For this review, take the finished solid that the model builds, in its own axes (mm). A direction names the side the tool comes from. Coordinates: 2 decimals unless noted, no trailing zeros. Loops run counter-clockwise (first coordinate to the right, second up) from the corner with the lowest first, then second, coordinate; pieces in that order, holes last. Notation, with made-up numbers: (87, -16) - (94, -16) arc R21 cw to (94, -1) - close; hole circle Ø7 at (57, -3.75). An arc over 180 degrees is marked (long way). One line per item, written item: value. Start each with the question number.
1. For faces 5 (the face through (-41.503, 6.12, -0.154)), 6 (the face through (-22.76, 3.595, 40.954)), 7 (the face through (42, 1.5, 7)), list the 3-axis set-ups (+Z, -Z, +X, -X, +Y, -Y) from which the entire face can be reached by the end or side of a thin tool; tool diameter is ignored.
2. To check wall thickness, follow line 1 (Z direction, x = -22.5, y = 6.1); line 2 (Z direction, x = 0, y = 0.75). State the ranges of each line that lie inside material, in increasing order. Write a range as from..to.
3. Take a section at A-A, the plane z = 0. Count the separate pieces of the cut face and the enclosed holes in it, and give its area (3 significant figures).
4. Insertion check: pin 1 (7.5 mm diameter, centred on x = -45, z = 0, fed in from +Y); pin 2 (3 mm diameter, centred on x = 25.5, y = 9, fed in from +Z); pin 3 (3.5 mm diameter, centred on x = -21, z = -39.5, fed in from +Y). Each pin has a flat end and moves straight along its axis. Give the tip position at first contact, or say it passes through.
5. Take a section at C-C, the plane x = 0. State the section outline as (y, z) points.
6. Take a section at D-D, the plane z = -12. State the section outline as (x, y) points, and give its area (3 significant figures).
7. The part is to be moulded in two halves that separate along Z. For faces 1 (the face through (-34, 6.5, -21)), 2 (the face through (-51, 4, 0)), 3 (the face through (43, 4, 0)), 4 (the face through (20, 5.75, -40)), say which applies: released by +Z, released by -Z, zero draft, split by the parting line, or undercut.
8. Take a section at B-B, the plane x = 45. State the section outline as (y, z) points, and give its area (3 significant figures).
```python
from build123d import *

# Parameters (mm, degrees)
EXTRUDE_1_DEPTH          = 5
PATTERN_CIRCULAR_1_COUNT = 6


with BuildPart() as part:
    # 草圖1 → 旋轉1 (revolve)
    with BuildSketch(Plane.XY):
        with BuildLine():
            Line((39.811273529, 6.5), (47.5, 6.5))
            Line((47.5, 6.5), (47.5, 1.5))
            Line((47.5, 1.5), (42, 1.5))
            Line((42, 1.5), (42, 0))
            Line((42, 0), (40, 0))
            Line((40, 0), (40, 0.927925359))
            ThreePointArc((40, 0.927925359), (22.903465984, 17.291823131), (0, 23.25))
            Line((0, 23.25), (0, 26.25))
            ThreePointArc((0, 26.25), (22.220486043, 21.041182168), (39.811273529, 6.5))
        make_face()
    revolve(axis=Axis((0, 0, 0), (0, 1, 0)))

    # 草圖3 → 填料-伸長1 (add)
    with BuildSketch(Plane(origin=(0, 6.5, 0), x_dir=(1, 0, 0), z_dir=(0, 1, 0))):
        with BuildLine():
            ThreePointArc((44.6, 5.986651819), (51, 0), (44.6, -5.986651819))
            ThreePointArc((44.6, -5.986651819), (45, 0), (44.6, 5.986651819))
        make_face()
        with BuildLine():
            ThreePointArc((27.484592559, -35.631407099), (25.5, -44.167295593), (17.115407441, -41.618058918))
            ThreePointArc((17.115407441, -41.618058918), (22.5, -38.97114317), (27.484592559, -35.631407099))
        make_face()
        with BuildLine():
            ThreePointArc((-17.115407441, -41.618058918), (-25.5, -44.167295593), (-27.484592559, -35.631407099))
            ThreePointArc((-27.484592559, -35.631407099), (-22.5, -38.97114317), (-17.115407441, -41.618058918))
        make_face()
        with BuildLine():
            ThreePointArc((-44.6, -5.986651819), (-51, 0), (-44.6, 5.986651819))
            ThreePointArc((-44.6, 5.986651819), (-45, 0), (-44.6, -5.986651819))
        make_face()
        with BuildLine():
            ThreePointArc((-27.484592559, 35.631407099), (-25.5, 44.167295593), (-17.115407441, 41.618058918))
            ThreePointArc((-17.115407441, 41.618058918), (-22.5, 38.97114317), (-27.484592559, 35.631407099))
        make_face()
        with BuildLine():
            ThreePointArc((17.115407441, 41.618058918), (25.5, 44.167295593), (27.484592559, 35.631407099))
            ThreePointArc((27.484592559, 35.631407099), (22.5, 38.97114317), (17.115407441, 41.618058918))
        make_face()
    extrude(amount=-EXTRUDE_1_DEPTH)

    # 草圖5 → 除料-旋轉1 (revolve, cut)
    with BuildSketch(Plane.XY):
        Polygon((48.5, 6.5), (48.5, 5.75), (47, 5.75), (47, 1.5), (45, 1.5), (45, 6.5), align=None)
    cut_revolve_1 = revolve(axis=Axis((45, 6.5, 0), (0, -1, 0)), mode=Mode.SUBTRACT)

    # 環狀複製排列1: 除料-旋轉1 ×6 about axis
    pattern_circular_1_axis = Axis((0, 0, 0), (0, 1, 0))
    for i in range(1, PATTERN_CIRCULAR_1_COUNT):
        add(cut_revolve_1.rotate(pattern_circular_1_axis, i * 360 / PATTERN_CIRCULAR_1_COUNT), mode=Mode.SUBTRACT)


solid = part.part
```
Solutions:
1. face 5: +Y
1. face 6: +Y, -Y
1. face 7: -Y
2. line 1: -44.97..-42.47, -35.47..-28.49, 28.49..35.47, 42.47..44.97
2. line 2: -42..-40, 40..42
3. separate pieces: 3
3. enclosed holes: 0
3. area: 354 mm2
4. pin 1: y = 6.5
4. pin 2: z = 29.99
4. pin 3: y = 5.75
5. outline: (0, -42) - (1.5, -42) - (1.5, -47.5) - (6.5, -47.5) - (6.5, -39.81) arc R50 ccw to (6.5, 39.81) - (6.5, 47.5) - (1.5, 47.5) - (1.5, 42) - (0, 42) - (0, 40) - (0.93, 40) arc R47 cw to (0.93, -40) - (0, -40) - close
6. outline: (-45.96, 1.5) - (-40.25, 1.5) - (-40.25, 0) - (-38.16, 0) - (-38.16, 0.93) arc R45.44 cw to (38.16, 0.93) - (38.16, 0) - (40.25, 0) - (40.25, 1.5) - (45.96, 1.5) - (45.96, 6.5) - (37.96, 6.5) arc R48.54 ccw to (-37.96, 6.5) - (-45.96, 6.5) - close
6. area: 360 mm2
7. face 1: zero draft
7. face 2: split by the parting line
7. face 3: undercut
7. face 4: undercut
8. outline: (1.5, -15.21) - (6.5, -15.21) - (6.5, -3.5) - (5.75, -3.5) - (5.75, -2) - (1.5, -2) - close; (1.5, 2) - (5.75, 2) - (5.75, 3.5) - (6.5, 3.5) - (6.5, 15.21) - (1.5, 15.21) - close
8. area: 130 mm2
